Design review of the part built by this model. Coordinates are the model's own, in mm. Face numbers are marked on the shaded views. A direction names the side the tool comes from. Round coordinates to 2 decimals unless told otherwise and drop trailing zeros. Order: outer loops, then holes, each group sorted by start corner. A loop starts at its lowest first (then second) coordinate and runs counter-clockwise, first axis right, second up. Notation, with made-up numbers: M 41.5,64 L 62.5,64 A16 ccw 62.5,95 Z; hole C 82.25,17.5 d10. An arc over 180 degrees is marked long. Use a Markdown table: item, result. Add a question column.
(1) Take a section at C-C (z = 6). Count the separate pieces of the cut face and the enclosed holes in it, then the cut area to 3 significant figures.
(2) Take a section at D-D (z = 45). Write out the cut boundary in (x, y), then the cut area to 3 significant figures.
(3) To check wall thickness, follow probe 1 along Z at (x, y) = (24.5, -17); probe 2 along Z at (x, y) = (15, -5); probe 3 along X at (y, z) = (-18, 16.5). State the ranges of each line that lie inside material, in increasing order. Write a range as from..to.
(4) Take a section at B-B (x = 0). Write out the cut boundary in (y, z), then the cut area to 4 significant figures.
(5) Take a section at A-A (z = 54). Write out the cut boundary in (x, y), then the cut area to 3 significant figures.
(6) The part is to be moulded in two halves that separate along X. For the marked faces 4, 5 and 6, say which applies: released by +X, released by -X, zero draft, split by the parting line, or undercut.
(7) For pin 1 (1 mm diameter, centred on x = 0, y = -20.5, fed in from -Z); pin 2 (6.5 mm diameter, centred on x = 4.5, y = -14, fed in from +Z); pin 3 (3 mm diameter, centred on y = -23.5, z = 57, fed in from -X), all flat-tipped, find the tip position at first contact; note any pin that passes through.
(8) Machinability: for the marked faces 1, 2 and 3, which of the approach directions +Z, -Z, +X, -X, +Y, -Y give a long, thin tool a straight path to every point of the face, cutting with its end or side? Answer none if there is none.
```python
from build123d import *

# Parameters (mm, degrees)
SKETCH_1_R               = 2
SKETCH_1_R_2             = 1.25
EXTRUDE_1_DEPTH          = 10.5
SKETCH_2_R               = 1.25
SKETCH_2_R_2             = 2
EXTRUDE_2_DEPTH          = 5
SKETCH_3_R               = 3
CUT_EXTRUDE_1_DEPTH      = 3.5
CHAMFER_1_SIZE           = 2
EXTRUDE_3_DEPTH          = 52
CUT_EXTRUDE_2_DEPTH      = 1
CUT_EXTRUDE_2_DEPTH_BACK = 53
SKETCH_7_R               = 21
CUT_EXTRUDE_4_DEPTH      = 43.5
CUT_EXTRUDE_4_DEPTH_BACK = 10.5
SKETCH_8_R               = 1.5
CUT_EXTRUDE_5_DEPTH      = 43.5000001
CUT_EXTRUDE_5_DEPTH_BACK = 10.5000001
SKETCH_10_R              = 3
CUT_EXTRUDE_6_DEPTH      = 3.2
CUT_EXTRUDE_START        = 33
SKETCH_10_2_R            = 3
CUT_EXTRUDE_8_DEPTH      = 3.2


with BuildPart() as part:
    # 草图1 → 凸台-拉伸1 (new body)
    with BuildSketch(Plane.XY):
        with BuildLine():
            ThreePointArc((-6.500553872, 18.384580478), (-18.384580478, -6.500553872), (6.500553872, -18.384580478))
            ThreePointArc((6.500553872, -18.384580478), (18.384580478, 6.500553872), (-6.500553872, 18.384580478))
        make_face()
        with Locations((-4.050345105, 11.455007836)):
            Circle(SKETCH_1_R, mode=Mode.SUBTRACT)
        with Locations((8.772394705, 10.261339637)):
            Circle(SKETCH_1_R_2, mode=Mode.SUBTRACT)
        with Locations((11.945500339, -2.219802163)):
            Circle(SKETCH_1_R, mode=Mode.SUBTRACT)
        with Locations((4.50038345, -12.727786485)):
            Circle(SKETCH_1_R_2, mode=Mode.SUBTRACT)
        with Locations((-7.895155235, -9.235205673)):
            Circle(SKETCH_1_R, mode=Mode.SUBTRACT)
        with Locations((-13.272778155, 2.466446848)):
            Circle(SKETCH_1_R_2, mode=Mode.SUBTRACT)
    extrude(amount=EXTRUDE_1_DEPTH)

    # 草图2 → 凸台-拉伸2 (add)
    with BuildSketch(Plane.XY.offset(10.5)):
        with BuildLine():
            Line((20, -26), (-20, -26))
            ThreePointArc((-20, -26), (-24.242640687, -24.242640687), (-26, -20))
            Line((-26, -20), (-26, 20))
            ThreePointArc((-26, 20), (-24.242640687, 24.242640687), (-20, 26))
            Line((-20, 26), (20, 26))
            ThreePointArc((20, 26), (24.242640687, 24.242640687), (26, 20))
            Line((26, 20), (26, -20))
            ThreePointArc((26, -20), (24.242640687, -24.242640687), (20, -26))
        make_face()
        with Locations((4.50038345, -12.727786485)):
            Circle(SKETCH_2_R, mode=Mode.SUBTRACT)
        with Locations((-7.895155235, -9.235205673)):
            Circle(SKETCH_2_R_2, mode=Mode.SUBTRACT)
        with Locations((-13.272778155, 2.466446848)):
            Circle(SKETCH_2_R, mode=Mode.SUBTRACT)
        with Locations((-4.050345105, 11.455007836)):
            Circle(SKETCH_2_R_2, mode=Mode.SUBTRACT)
        with Locations((11.945500339, -2.219802163)):
            Circle(SKETCH_2_R_2, mode=Mode.SUBTRACT)
        with Locations((8.772394705, 10.261339637)):
            Circle(SKETCH_2_R, mode=Mode.SUBTRACT)
    extrude(amount=EXTRUDE_2_DEPTH)

    # 草图3 → 切除-拉伸1 (cut)
    with BuildSketch(Plane.XY.offset(15.5)):
        with Locations((4.50038345, -12.727786485)):
            Circle(SKETCH_3_R)
        with Locations((-13.272778155, 2.466446848)):
            Circle(SKETCH_3_R)
        with Locations((8.772394705, 10.261339637)):
            Circle(SKETCH_3_R)
    extrude(amount=-CUT_EXTRUDE_1_DEPTH, mode=Mode.SUBTRACT)

    # 倒角1
    chamfer_1_edges = [part.edges().sort_by_distance(p)[0] for p in [
        (6.500553872, -18.384580478, 10.5),
    ]]
    chamfer(chamfer_1_edges, length=CHAMFER_1_SIZE)

    # 草图4 → 凸台-拉伸3 (add)
    with BuildSketch(Plane.XY.offset(15.5)):
        with BuildLine():
            Line((-16.5, -26), (-20, -26))
            ThreePointArc((-20, -26), (-24.242640687, -24.242640687), (-26, -20))
            Line((-26, -20), (-26, 20))
            ThreePointArc((-26, 20), (-24.242640687, 24.242640687), (-20, 26))
            Line((-20, 26), (-16.5, 26))
            Line((-16.5, 26), (-16.5, -26))
        make_face()
        with BuildLine():
            Line((16.5, 26), (20, 26))
            ThreePointArc((20, 26), (24.242640687, 24.242640687), (26, 20))
            Line((26, 20), (26, -20))
            ThreePointArc((26, -20), (24.242640687, -24.242640687), (20, -26))
            Line((20, -26), (16.5, -26))
            Line((16.5, -26), (16.5, 26))
        make_face()
    extrude(amount=EXTRUDE_3_DEPTH)

    # 草图5 → 切除-拉伸2 (cut, two sides)
    with BuildSketch(Plane.ZY.offset(26)) as cut_extrude_2_sk:
        with BuildLine():
            Line((61.5, -26), (67.5, -26))
            Line((67.5, -26), (67.5, -20))
            ThreePointArc((67.5, -20), (65.742640687, -24.242640687), (61.5, -26))
        make_face()
        with BuildLine():
            Line((61.5, 26), (67.5, 26))
            Line((67.5, 26), (67.5, 20))
            ThreePointArc((67.5, 20), (65.742640687, 24.242640687), (61.5, 26))
        make_face()
    extrude(amount=CUT_EXTRUDE_2_DEPTH, mode=Mode.SUBTRACT)
    extrude(cut_extrude_2_sk.sketch, amount=-CUT_EXTRUDE_2_DEPTH_BACK, mode=Mode.SUBTRACT)

    # 草图7 → 切除-拉伸4 (cut, two sides)
    with BuildSketch(Plane(origin=(-16.5, 0, 0), x_dir=(0, 0, -1), z_dir=(1, 0, 0))) as cut_extrude_4_sk:
        with Locations((-42, 0)):
            Circle(SKETCH_7_R)
    extrude(amount=CUT_EXTRUDE_4_DEPTH, mode=Mode.SUBTRACT)
    extrude(cut_extrude_4_sk.sketch, amount=-CUT_EXTRUDE_4_DEPTH_BACK, mode=Mode.SUBTRACT)

    # 草图8 → 切除-拉伸5 (cut, two sides)
    with BuildSketch(Plane(origin=(-16.5, 0, 0), x_dir=(0, 0, -1), z_dir=(1, 0, 0))) as cut_extrude_5_sk:
        with Locations((-57.969331475, -22.388176617)):
            Circle(SKETCH_8_R)
        with Locations((-19.611823383, -15.969331475)):
            Circle(SKETCH_8_R)
        with Locations((-26.030668525, 22.388176617)):
            Circle(SKETCH_8_R)
        with Locations((-64.388176617, 15.969331475)):
            Circle(SKETCH_8_R)
    extrude(amount=CUT_EXTRUDE_5_DEPTH, mode=Mode.SUBTRACT)
    extrude(cut_extrude_5_sk.sketch, amount=-CUT_EXTRUDE_5_DEPTH_BACK, mode=Mode.SUBTRACT)

    # 草图10 → 切除-拉伸6 (cut)
    with BuildSketch(Plane(origin=(-16.5, 0, 0), x_dir=(0, 0, -1), z_dir=(1, 0, 0))):
        with Locations((-64.388176617, 15.969331475)):
            Circle(SKETCH_10_R)
        with Locations((-26.030668525, 22.388176617)):
            Circle(SKETCH_10_R)
        with Locations((-19.611823383, -15.969331475)):
            Circle(SKETCH_10_R)
        with Locations((-57.969331475, -22.388176617)):
            Circle(SKETCH_10_R)
    extrude(amount=-CUT_EXTRUDE_6_DEPTH, mode=Mode.SUBTRACT)

    # 草图10<2> → 切除-拉伸8 (cut)
    with BuildSketch(Plane(origin=(-16.5, 0, 0), x_dir=(0, 0, -1), z_dir=(1, 0, 0)).offset(CUT_EXTRUDE_START)):
        with Locations((-64.388176617, 15.969331475)):
            Circle(SKETCH_10_2_R)
        with Locations((-26.030668525, 22.388176617)):
            Circle(SKETCH_10_2_R)
        with Locations((-19.611823383, -15.969331475)):
            Circle(SKETCH_10_2_R)
        with Locations((-57.969331475, -22.388176617)):
            Circle(SKETCH_10_2_R)
    extrude(amount=CUT_EXTRUDE_8_DEPTH, mode=Mode.SUBTRACT)


solid = part.part
```
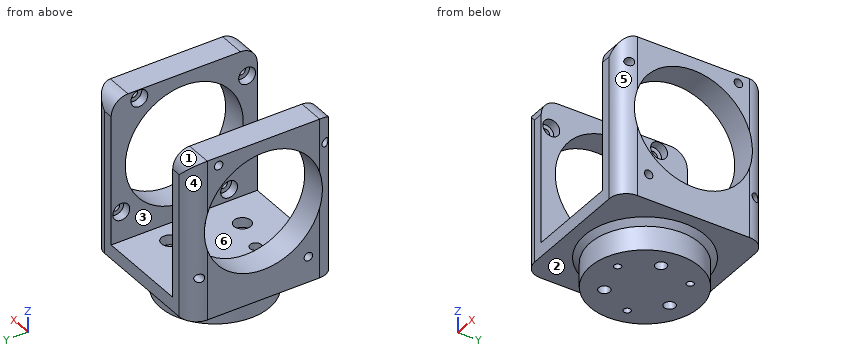
Verdict:
| question | item | result |
|---|---|---|
| 1 | separate pieces | 1 |
| 1 | enclosed holes | 6 |
| 1 | area | 1,140 mm^2 |
| 2 | outline | M -25.95,-20.78 A6 ccw -20,-26 L -16.5,-26 L -16.5,-20.78 Z; M -25.95,20.78 L -16.5,20.78 L -16.5,26 L -20,26 A6 ccw Z; M 16.5,-26 L 20,-26 A6 ccw 25.95,-20.78 L 16.5,-20.78 Z; M 16.5,20.78 L 25.95,20.78 A6 ccw 20,26 L 16.5,26 Z |
| 2 | area | 167 mm^2 |
| 3 | probe 1 | z = 10.5..18.52, 20.7..29.67, 54.33..67.5 |
| 3 | probe 2 | z = 0..15.5 |
| 3 | probe 3 | x = -26..-16.5, 16.5..26 |
| 4 | outline | M -26,10.5 L -21.5,10.5 L -19.5,8.5 L -19.5,0 L 19.5,0 L 19.5,8.5 L 21.5,10.5 L 26,10.5 L 26,15.5 L -26,15.5 Z |
| 4 | area | 673.5 mm^2 |
| 5 | outline | M -26,-20 A6 ccw -20,-26 L -16.5,-26 L -16.5,-17.23 L -26,-17.23 Z; M -26,17.23 L -16.5,17.23 L -16.5,26 L -20,26 A6 ccw -26,20 Z; M 16.5,-26 L 20,-26 A6 ccw 26,-20 L 26,-17.23 L 16.5,-17.23 Z; M 16.5,17.23 L 26,17.23 L 26,20 A6 ccw 20,26 L 16.5,26 Z |
| 5 | area | 302 mm^2 |
| 6 | face 4 | released by -X |
| 6 | face 5 | released by +X |
| 6 | face 6 | undercut |
| 7 | pin 1 | stops at z = 9 |
| 7 | pin 2 | stops at z = 15.5 |
| 7 | pin 3 | stops at x = -25.63 |
| 8 | face 1 | +Z, +X, -X, +Y |
| 8 | face 2 | -Z |
| 8 | face 3 | +Z, +Y, -Y |
